Can you work these out from the drawing? Everything is in mm from the part's minimum corner. Give positions to 0.01 mm unless a question says otherwise; leave off trailing zeros. Write each loop counter-clockwise with the first axis right and the second up, starting at its lowest first coordinate (ties: lowest second). Pieces come first, ordered by that corner, then holes. Notation, with made-up numbers: (79.25, -20) - (120.25, -20) arc R19 ccw to (120.25, -9) - close; hole circle Ø4 at (-26.75, 0). An arc over 180 degrees is marked (long way). Answer in a Markdown table with one row per item.
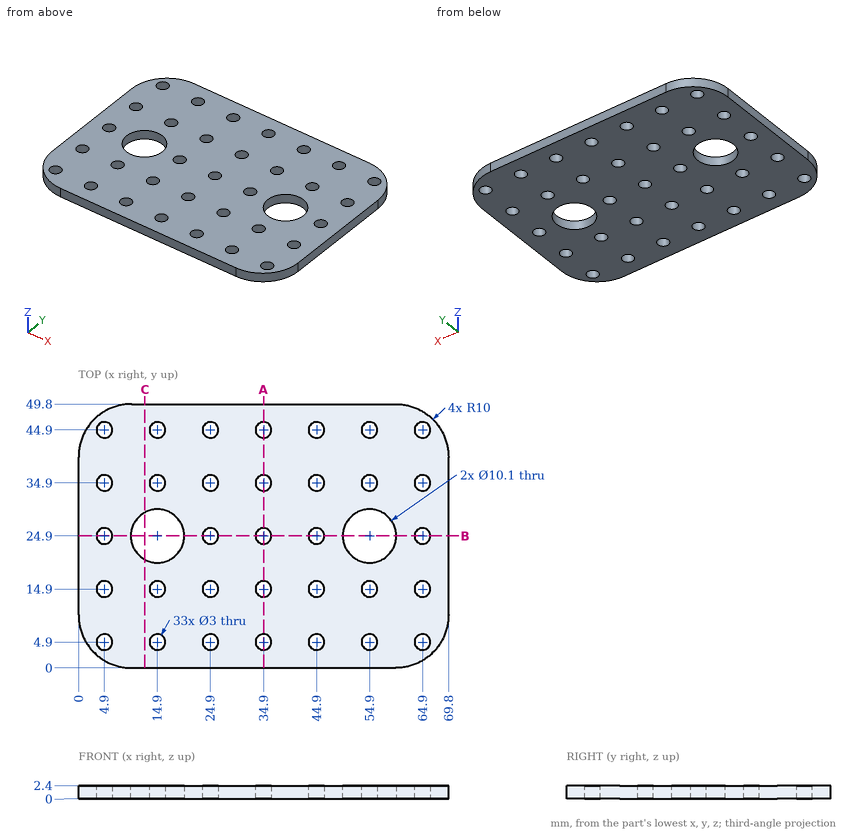
1) If I drill on line 1 (Y direction, x = 24.9, z = 0.6); line 2 (X direction, y = 26.5, z = 2); line 3 (X direction, y = 21.5, z = 0.6), over which ranges is the centre line in solid material (lowest first)?
Check values:
| item | result |
|---|---|
| line 1 | y = 0 to 3.4, 6.4 to 13.4, 16.4 to 23.4, 26.4 to 33.4, 36.4 to 43.4, 46.4 to 49.8 |
| line 2 | x = 0 to 10.11, 19.69 to 50.11, 59.69 to 69.8 |
| line 3 | x = 0 to 11.17, 18.63 to 51.17, 58.63 to 69.8 |
2) Imagine slicing it at C-C (x = 12.5). List the corners of the cut face in (y, z) for me, then the cut area to 3 significant figures.
Check values:
| item | result |
|---|---|
| outline | (0, 0) - (20.46, 0) - (20.46, 2.4) - (0, 2.4) - close; (29.34, 0) - (49.8, 0) - (49.8, 2.4) - (29.34, 2.4) - close |
| area | 98.2 mm2 |
3) Imagine slicing it at A-A (x = 34.9). List the corners of the cut face in (y, z) for me, then the cut area to 3 significant figures.
Check values:
| item | result |
|---|---|
| outline | (0, 0) - (3.4, 0) - (3.4, 2.4) - (0, 2.4) - close; (6.4, 0) - (13.4, 0) - (13.4, 2.4) - (6.4, 2.4) - close; (16.4, 0) - (23.4, 0) - (23.4, 2.4) - (16.4, 2.4) - close; (26.4, 0) - (33.4, 0) - (33.4, 2.4) - (26.4, 2.4) - close; (36.4, 0) - (43.4, 0) - (43.4, 2.4) - (36.4, 2.4) - close; (46.4, 0) - (49.8, 0) - (49.8, 2.4) - (46.4, 2.4) - close |
| area | 83.5 mm2 |
4) Will this pin go through, and if not, where does the flat tip stop? P1, Ø2.5, axis at x = 14.9, y = 14.9, coming from the +Z side.
Check values:
| item | result |
|---|---|
| P1 | passes through |
5) Imagine slicing it at B-B (y = 24.9). State how many separate pieces and enclosed holes the cut face has, then the cut area to 3 significant figures.
Check values:
| item | result |
|---|---|
| separate pieces | 8 |
| enclosed holes | 0 |
| area | 83.0 mm2 |
